Check sheet for the modelled part. Datum: model origin and axes. Units: mm. A direction names the side the tool comes from. Coordinates: 2 decimals unless noted, no trailing zeros. Order: outer loops, then holes, each group sorted by start corner. A loop starts at its lowest first (then second) coordinate and runs counter-clockwise, first axis right, second up.
from build123d import *

# Parameters (mm, degrees)
F1_DEPTH = 1.05
F2_R     = 0.396875
F4_DEPTH = 2.101


with BuildPart() as f1:
    # F0 (on Top) → F1 (new body, symmetric)
    with BuildSketch(Plane.XY):
        with BuildLine():
            ThreePointArc((1.2711994223, -0.5554208485), (0, -0.2898326497), (-1.2711994223, -0.5554208485))
            Line((-1.2711994223, -0.5554208485), (-8.9961994223, -3.930678876))
            ThreePointArc((-8.9961994223, -3.930678876), (-10.381753956, -5.1016191022), (-10.9, -6.8400906772))
            Line((-10.9, -6.8400906772), (-10.9, -17.9896228211))
            ThreePointArc((-10.9, -17.9896228211), (-10.381753956, -19.7280943961), (-8.9961994223, -20.8990346223))
            Line((-8.9961994223, -20.8990346223), (-7.3400002889, -21.6226720877))
            ThreePointArc((-7.3400002889, -21.6226720877), (-6.647223022, -22.2081422008), (-6.3881, -23.0773779883))
            Line((-6.3881, -23.0773779883), (-6.3881, -24.4198326497))
            Line((-6.3881, -24.4198326497), (-4.2672, -24.4198326497))
            Line((-4.2672, -24.4198326497), (-4.2672, -52.3598326497))
            Line((-4.2672, -52.3598326497), (4.2672, -52.3598326497))
            Line((4.2672, -52.3598326497), (4.2672, -24.4198326497))
            Line((4.2672, -24.4198326497), (6.3881, -24.4198326497))
            Line((6.3881, -24.4198326497), (6.3881, -23.0773779883))
            ThreePointArc((6.3881, -23.0773779883), (6.647223022, -22.2081422008), (7.3400002889, -21.6226720877))
            Line((7.3400002889, -21.6226720877), (8.9961994223, -20.8990346223))
            ThreePointArc((8.9961994223, -20.8990346223), (10.381753956, -19.7280943961), (10.9, -17.9896228211))
            Line((10.9, -17.9896228211), (10.9, -6.8400906772))
            ThreePointArc((10.9, -6.8400906772), (10.381753956, -5.1016191022), (8.9961994223, -3.930678876))
            Line((8.9961994223, -3.930678876), (1.2711994223, -0.5554208485))
        make_face()
    extrude(amount=F1_DEPTH, both=True)

    # F2
    f2_edges = [f1.edges().sort_by_distance(p)[0] for p in [
        (6.3881, -24.419833, 0),
        (-6.3881, -24.419833, 0),
    ]]
    fillet(f2_edges, radius=F2_R)

    # F3 (on face) → F4 (cut, through all)
    with BuildSketch(Plane.XY.offset(1.05)):
        with BuildLine():
            ThreePointArc((0.2542398845, -2.8829502894), (0, -2.8298326497), (-0.2542398845, -2.8829502894))
            Line((-0.2542398845, -2.8829502894), (-4.6036733755, -4.7833335005))
            ThreePointArc((-4.6036733755, -4.7833335005), (-4.7192112161, -4.9283315767), (-4.6645399135, -5.10548824))
            Line((-4.6645399135, -5.10548824), (-0.1403165019, -9.6297116516))
            ThreePointArc((-0.1403165019, -9.6297116516), (0, -9.6878326497), (0.1403165019, -9.6297116516))
            Line((0.1403165019, -9.6297116516), (4.6645399135, -5.10548824))
            ThreePointArc((4.6645399135, -5.10548824), (4.7192112161, -4.9283315767), (4.6036733755, -4.7833335005))
            Line((4.6036733755, -4.7833335005), (0.2542398845, -2.8829502894))
        make_face()
        with BuildLine():
            ThreePointArc((-7.4941261238, -6.0462492082), (-8.1242947921, -6.5788084291), (-8.36, -7.3694884715))
            Line((-8.36, -7.3694884715), (-8.36, -11.7753951497))
            ThreePointArc((-8.36, -11.7753951497), (-8.3018790019, -11.9157116516), (-8.1615625, -11.9738326497))
            Line((-8.1615625, -11.9738326497), (-1.867368456, -11.9738326497))
            ThreePointArc((-1.867368456, -11.9738326497), (-1.6840361113, -11.8513338933), (-1.7270519541, -11.6350786478))
            Line((-1.7270519541, -11.6350786478), (-7.274359658, -6.0877709439))
            ThreePointArc((-7.274359658, -6.0877709439), (-7.3778359984, -6.0330996413), (-7.4941261238, -6.0462492082))
        make_face()
        with BuildLine():
            Line((8.36, -11.7753951497), (8.36, -7.3694884715))
            ThreePointArc((8.36, -7.3694884715), (8.1242947921, -6.5788084291), (7.4941261238, -6.0462492082))
            ThreePointArc((7.4941261238, -6.0462492082), (7.3778359984, -6.0330996413), (7.274359658, -6.0877709439))
            Line((7.274359658, -6.0877709439), (1.7270519541, -11.6350786478))
            ThreePointArc((1.7270519541, -11.6350786478), (1.6840361113, -11.8513338933), (1.867368456, -11.9738326497))
            Line((1.867368456, -11.9738326497), (8.1615625, -11.9738326497))
            ThreePointArc((8.1615625, -11.9738326497), (8.3018790019, -11.9157116516), (8.36, -11.7753951497))
        make_face()
    extrude(amount=-F4_DEPTH, mode=Mode.SUBTRACT)


solid = f1.part
(1) Cross-section at C-C (x = -5.5). Enter the section's corners in (y, z), and give its area (3 significant figures).
Filled in:
outline: (-24.42, -1.05) - (-11.97, -1.05) - (-11.97, 1.05) - (-24.42, 1.05) - close; (-7.86, -1.05) - (-2.4, -1.05) - (-2.4, 1.05) - (-7.86, 1.05) - close
area: 37.6 mm2
(2) Cross-section at A-A (x = 2.5). Enter the section's corners in (y, z), and give its area (3 significant figures).
Filled in:
outline: (-52.36, -1.05) - (-11.97, -1.05) - (-11.97, 1.05) - (-52.36, 1.05) - close; (-10.86, -1.05) - (-7.27, -1.05) - (-7.27, 1.05) - (-10.86, 1.05) - close; (-3.86, -1.05) - (-1.09, -1.05) - (-1.09, 1.05) - (-3.86, 1.05) - close
area: 98.2 mm2
(3) Thickness scan on probe 1 along Y at (x, z) = (-2.5, -0.65); probe 2 along Y at (x, z) = (-1.75, 0.75); probe 3 along X at (y, z) = (-27.5, 0.8). Record the ranges inside material, lowest first.
Filled in:
probe 1: y = -52.36 to -11.97, -10.86 to -7.27, -3.86 to -1.09
probe 2: y = -52.36 to -11.94, -11.61 to -8.02, -3.54 to -0.76
probe 3: x = -4.27 to 4.27
(4) Cross-section at D-D (y = -43.5). Enter the section's corners in (x, z).
Filled in:
outline: (-4.27, -1.05) - (4.27, -1.05) - (4.27, 1.05) - (-4.27, 1.05) - close
(5) Cross-section at B-B (z = -0.6). Count the separate pieces of the cut face and the enclosed holes in it, and give its area (3 significant figures).
Filled in:
separate pieces: 1
enclosed holes: 3
area: 605 mm2
(6) Release check for a two-part mould opening along X. For faces 6 (the cylindrical face through (0.02, -0.29, 0.01)), 7 (the flat face through (8.157, -21.266, 0.015)), 8 (the flat face through (-8.18, -21.256, 0.015)), 9 (the flat face through (2.459, -3.846, 0.015)) record: +X half, -X half, draft (parallel to the pull), parting line (faces both ways), or undercut.
Filled in:
face 6: parting line
face 7: +X half
face 8: -X half
face 9: undercut
(7) Tool access check on faces 1 (the flat face through (5.188, -2.267, 0.015)), 2 (the flat face through (-4.267, -38, 0)), 3 (the flat face through (0, -20, 1.05)), 4 (the cylindrical face through (-8.12, -6.57, 0.01)), 5 (the flat face through (4.267, -39, 0)). Record the directions out of +Z, -Z, +X, -X, +Y, -Y that give a thin tool (end or side, any length) a straight path to the whole face; none if there is none.
Filled in:
face 1: +Z, -Z, +X, +Y
face 2: +Z, -Z, -X, -Y
face 3: +Z, +X, -X, +Y, -Y
face 4: +Z, -Z
face 5: +Z, -Z, +X, -Y
(8) Go/stop test with flat-tipped pins: P1, Ø1, axis at y = -36, z = 0, coming from the -X side; P2, Ø0.8, axis at y = -23.5, z = 0, coming from the +X side; P3, Ø1, axis at y = -31.5, z = 0, coming from the +X side. Record where each tip stops, or that it passes through.
Filled in:
P1: stops at x = -4.27
P2: stops at x = 6.39
P3: stops at x = 4.27
